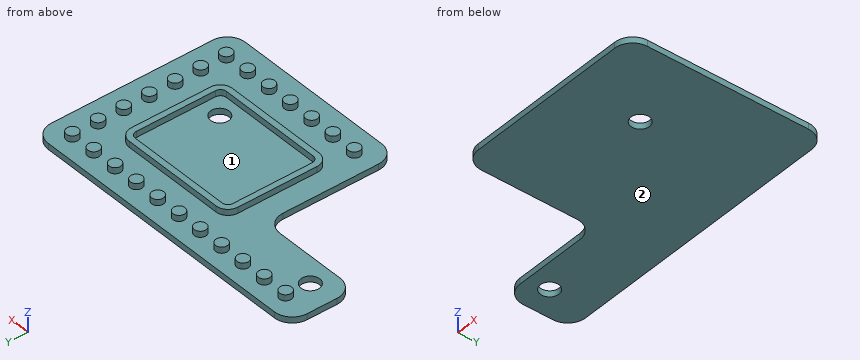
from build123d import *

# Parameters (mm, degrees)
BOSS_EXTRUDE1_DEPTH = 1
SKETCH2_R           = 1
BOSS_EXTRUDE2_DEPTH = 1
FILLET1_R           = 3
CUT_EXTRUDE1_REACH  = 3
SKETCH3_R           = 1.55


with BuildPart() as part:
    # Sketch1 → Boss-Extrude1 (new body)
    with BuildSketch(Plane.XY):
        Polygon((-8, 5), (-8, 38), (-59.580513121, 38), (-59.580513121, 27), (-41.5, 27), (-41.5, 5), align=None)
    extrude(amount=BOSS_EXTRUDE1_DEPTH)

    # Sketch2 → Boss-Extrude2 (add)
    with BuildSketch(Plane.XY.offset(1)):
        with Locations((-12, 9)):
            Circle(SKETCH2_R)
        with Locations((-12, 13.3)):
            Circle(SKETCH2_R)
        with Locations((-12, 17.6)):
            Circle(SKETCH2_R)
        with Locations((-12, 21.9)):
            Circle(SKETCH2_R)
        with Locations((-12, 26.2)):
            Circle(SKETCH2_R)
        with Locations((-12, 30.5)):
            Circle(SKETCH2_R)
        with Locations((-12, 34.8)):
            Circle(SKETCH2_R)
        with Locations((-16.3, 9)):
            Circle(SKETCH2_R)
        with Locations((-20.6, 9)):
            Circle(SKETCH2_R)
        with Locations((-24.9, 9)):
            Circle(SKETCH2_R)
        with Locations((-29.2, 9)):
            Circle(SKETCH2_R)
        with Locations((-33.5, 9)):
            Circle(SKETCH2_R)
        with Locations((-37.8, 9)):
            Circle(SKETCH2_R)
        with Locations((-16.3, 34.8)):
            Circle(SKETCH2_R)
        with Locations((-20.6, 34.8)):
            Circle(SKETCH2_R)
        with Locations((-24.9, 34.8)):
            Circle(SKETCH2_R)
        with Locations((-29.2, 34.8)):
            Circle(SKETCH2_R)
        with Locations((-33.5, 34.8)):
            Circle(SKETCH2_R)
        with Locations((-37.8, 34.8)):
            Circle(SKETCH2_R)
        with Locations((-42.1, 34.8)):
            Circle(SKETCH2_R)
        with Locations((-46.4, 34.8)):
            Circle(SKETCH2_R)
        with Locations((-50.7, 34.8)):
            Circle(SKETCH2_R)
        with Locations((-55, 34.8)):
            Circle(SKETCH2_R)
        with BuildLine():
            Line((-35.8, 30.5), (-18.3, 30.5))
            ThreePointArc((-18.3, 30.5), (-16.885786438, 29.914213562), (-16.3, 28.5))
            Line((-16.3, 28.5), (-16.3, 15.236025644))
            ThreePointArc((-16.3, 15.236025644), (-16.885786438, 13.821812082), (-18.3, 13.236025644))
            Line((-18.3, 13.236025644), (-35.8, 13.236025644))
            ThreePointArc((-35.8, 13.236025644), (-37.214213562, 13.821812082), (-37.8, 15.236025644))
            Line((-37.8, 15.236025644), (-37.8, 28.5))
            ThreePointArc((-37.8, 28.5), (-37.214213562, 29.914213562), (-35.8, 30.5))
        make_face()
        with BuildLine():
            Line((-35.8, 29.5), (-18.3, 29.5))
            ThreePointArc((-18.3, 29.5), (-17.592893219, 29.207106781), (-17.3, 28.5))
            Line((-17.3, 28.5), (-17.3, 15.236025644))
            ThreePointArc((-17.3, 15.236025644), (-17.592893219, 14.528918863), (-18.3, 14.236025644))
            Line((-18.3, 14.236025644), (-35.8, 14.236025644))
            ThreePointArc((-35.8, 14.236025644), (-36.507106781, 14.528918863), (-36.8, 15.236025644))
            Line((-36.8, 15.236025644), (-36.8, 28.5))
            ThreePointArc((-36.8, 28.5), (-36.507106781, 29.207106781), (-35.8, 29.5))
        make_face(mode=Mode.SUBTRACT)
    extrude(amount=BOSS_EXTRUDE2_DEPTH)

    # Fillet1
    fillet1_edges = [part.edges().sort_by_distance(p)[0] for p in [
        (-41.5, 5, 0.5),
        (-41.5, 27, 0.5),
        (-59.580513121, 27, 0.5),
        (-59.580513121, 38, 0.5),
        (-8, 38, 0.5),
        (-8, 5, 0.5),
    ]]
    fillet(fillet1_edges, radius=FILLET1_R)

    # Sketch3 → Cut-Extrude1 (cut, up to next)
    with BuildSketch(Plane.XY.offset(1), mode=Mode.PRIVATE) as cut_extrude1_sk1:
        with Locations((-20.677552724, 17.314204089)):
            Circle(SKETCH3_R)
    cut_extrude1_tool1 = extrude(cut_extrude1_sk1.sketch, amount=-CUT_EXTRUDE1_REACH, mode=Mode.PRIVATE) & part.part
    add(cut_extrude1_tool1.solids().sort_by_distance((-20.677553, 17.314204, 1))[0], mode=Mode.SUBTRACT)
    # Sketch3 → Cut-Extrude1 (cut, up to next)
    with BuildSketch(Plane.XY.offset(1), mode=Mode.PRIVATE) as cut_extrude1_sk2:
        with Locations((-55, 30.651276125)):
            Circle(SKETCH3_R)
    cut_extrude1_tool2 = extrude(cut_extrude1_sk2.sketch, amount=-CUT_EXTRUDE1_REACH, mode=Mode.PRIVATE) & part.part
    add(cut_extrude1_tool2.solids().sort_by_distance((-55, 30.651276, 1))[0], mode=Mode.SUBTRACT)


solid = part.part
Source: CAD feature listing. Evaluate the final solid. Frame: model axes, mm. Face numbers are marked on the shaded views. Round coordinates to 2 decimals unless told otherwise and drop trailing zeros. Loops run counter-clockwise (first coordinate to the right, second up) from the corner with the lowest first, then second, coordinate; pieces in that order, holes last. Notation, with made-up numbers: (41.25, -35.5) - (99.25, -35.5) arc R27 ccw to (99.25, -9.5) - close; hole circle Ø1 at (40.5, 8.25). An arc over 180 degrees is marked (long way). Write item = value, one per line. Start each with the question number.
Item 1: Section query A-A on x = -55. Output: boundary loops of the cut face in (y, z).
Item 2: First-contact query: pin 1 Ø10 at (x, y) = (-36, 23) entering from -Z; pin 2 Ø0.5 at (x, z) = (-48, 0.5) entering from -Y; pin 3 Ø1.9 at (x, y) = (-20.68, 17.31) entering from -Z; pin 4 Ø1 at (y, z) = (12, 1) entering from -X. Flat tips, straight axial feed; report the tip coordinate or a pass-through.
Item 3: Material intervals for line 1 (Y direction, x = -25, z = 1.45); line 2 (Y direction, x = -55, z = 0.2); line 3 (Y direction, x = -31, z = 1.05), sorted ascending.
Item 4: Section query D-D on x = -42.1. Output: boundary loops of the cut face in (y, z), plus the area to 3 significant figures.
Item 5: Mould query, pull axis X, two halves, no side actions, for the marked faces 1 and 2. Classes: released by +X, released by -X, zero draft, split by the parting line, or undercut.
Item 6: Section query C-C on z = 1.5. Count the separate pieces of the cut face and the enclosed holes in it, plus the area to 3 significant figures.
Results list:
q1.outline = (27, 0) - (29.1, 0) - (29.1, 1) - (27, 1) - close; (32.2, 0) - (38, 0) - (38, 1) - (35.8, 1) - (35.8, 2) - (33.8, 2) - (33.8, 1) - (32.2, 1) - close
q2.pin_1 = 0
q2.pin_2 = 27
q2.pin_3 = through
q2.pin_4 = -41.5
q3.line_1 = 8.01 to 9.99, 13.24 to 14.24, 29.5 to 30.5, 33.81 to 35.79
q3.line_2 = 27 to 29.1, 32.2 to 38
q3.line_3 = 13.24 to 14.24, 29.5 to 30.5
q4.outline = (25.8, 0) - (38, 0) - (38, 1) - (35.8, 1) - (35.8, 2) - (33.8, 2) - (33.8, 1) - (25.8, 1) - close
q4.area = 14.2 mm²
q5.face_1 = undercut
q5.face_2 = zero draft
q6.separate_pieces = 24
q6.enclosed_holes = 1
q6.area = 143 mm²
